Autodesk Inventor part; units mm, degrees
ref_plane "YZ Plane" through (0, 0, 0) normal (1, 0, 0) x (0, 1, 0)
ref_plane "XZ Plane" through (0, 0, 0) normal (0, 1, 0) x (-1, 0, 0)
ref_plane "XY Plane" through (0, 0, 0) normal (0, 0, 1) x (1, 0, 0)
sketch "Sketch6" plane through (0, 0, 0) normal (0, 1, 0) x (-1, 0, 0)
  line L0 (407.1, -490) -> (-407.1, -490)
  line L1 (-407.1, -490) -> (-407.1, 490)
  line L2 (-407.1, 490) -> (407.1, 490)
  line L3 (407.1, 490) -> (407.1, -490)
  line L4 (407.1, -490) -> (-407.1, 490) construction
  line L5 (-407.1, -490) -> (407.1, 490) construction
  point P0 (0, 0)
  dimension "d52" = 814.2
  dimension "d53" = 980
extrude "Plate2" add sketch "Sketch6" along normal blind 0.5
sketch "Sketch11" plane through (406.6, 0, -490) normal (1, 0, 0) x (0, 1, 0)
  line L0 (0, 980) -> (0, 0)
  line L1 (0, 0) -> (10, 0)
  line L2 (10, 0) -> (10, 980)
  line L3 (10, 980) -> (0, 980)
edge flange "Flange2" height 10 angle 90 thickness 0.5 bend radius 0.5 thickness toward (1, 0, 0) relief tear relief width 0.5 relief depth 0.25 edges at (407.1, 0.5, 0) wall of the first edge with corners at (406.6, 0, 490) (406.6, 0, -490) (406.6, 10, -490) (406.6, 10, 490)
bend "Bend3"
corner "Corner3"
sketch "Sketch12" plane through (407.1, 9.5, -490) normal (0, 1, 0) x (-1, 0, 0)
  line L0 (0, 980) -> (0, 0)
  line L1 (0, 0) -> (10, 0)
  line L2 (10, 0) -> (10, 980)
  line L3 (10, 980) -> (0, 980)
edge flange "Flange3" height 10 angle 90 thickness 0.5 bend radius 0.5 thickness toward (0, 1, 0) relief tear relief width 0.5 relief depth 0.25 edges at (406.6, 10, 0) wall of the first edge with corners at (407.1, 9.5, 490) (407.1, 9.5, -490) (397.1, 9.5, -490) (397.1, 9.5, 490)
bend "Bend4"
corner "Corner4"
sketch "Sketch13" plane through (-406.6, 0, 490) normal (-1, 0, 0) x (0, -1, 0)
  line L0 (0, -980) -> (0, 0)
  line L1 (0, 0) -> (-10, 0)
  line L2 (-10, 0) -> (-10, -980)
  line L3 (-10, -980) -> (0, -980)
edge flange "Flange4" height 10 angle 90 thickness 0.5 bend radius 0.5 thickness toward (-1, 0, 0) relief tear relief width 0.5 relief depth 0.25 edges at (-407.1, 0.5, 0) wall of the first edge with corners at (-406.6, 0, -490) (-406.6, 0, 490) (-406.6, 10, 490) (-406.6, 10, -490)
bend "Bend5"
corner "Corner5"
sketch "Sketch14" plane through (-407.1, 9.5, 490) normal (0, 1, 0) x (-1, 0, 0)
  line L0 (0, -980) -> (0, 0)
  line L1 (0, 0) -> (-10, 0)
  line L2 (-10, 0) -> (-10, -980)
  line L3 (-10, -980) -> (0, -980)
edge flange "Flange5" height 10 angle 90 thickness 0.5 bend radius 0.5 thickness toward (0, 1, 0) relief tear relief width 0.5 relief depth 0.25 edges at (-406.6, 10, 0) wall of the first edge with corners at (-407.1, 9.5, -490) (-407.1, 9.5, 490) (-397.1, 9.5, 490) (-397.1, 9.5, -490)
bend "Bend6"
corner "Corner6"
fillet "Corner Round1" radius 4 1 edges at (397.1, 9.75, 490)
fillet "Corner Round2" radius 4 1 edges at (397.1, 9.75, -490)
fillet "Corner Round3" radius 4 1 edges at (-397.1, 9.75, -490)
fillet "Corner Round4" radius 4 1 edges at (-397.1, 9.75, 490)
equation "\"d52\" = ЖАБРЫ_базовая_ширина - ЖАБРЫ_шаг_листов"
equation "\"d53\" = ЖАБРЫ_базовая_длина_кор_лист"
equation "\"d54\" = Thickness"
equation "\"d84\" = BendReliefWidth"
equation "\"d85\" = BendReliefDepth"
equation "\"d86\" = MinimumRemnant"
equation "\"d87\" = TransitionRadius"
equation "\"d90\" = BendRadius"
equation "\"d91\" = CornerReliefSize"
equation "\"d92\" = GapSize"
equation "\"d93\" = JacobiRadiusSize"
equation "\"d94\" = BendReliefWidth"
equation "\"d95\" = BendReliefDepth"
equation "\"d96\" = MinimumRemnant"
equation "\"d97\" = TransitionRadius"
equation "\"d100\" = BendRadius"
equation "\"d101\" = CornerReliefSize"
equation "\"d102\" = GapSize"
equation "\"d103\" = JacobiRadiusSize"
equation "\"d104\" = BendReliefWidth"
equation "\"d105\" = BendReliefDepth"
equation "\"d106\" = MinimumRemnant"
equation "\"d107\" = TransitionRadius"
equation "\"d110\" = BendRadius"
equation "\"d111\" = CornerReliefSize"
equation "\"d112\" = GapSize"
equation "\"d113\" = JacobiRadiusSize"
equation "\"d114\" = BendReliefWidth"
equation "\"d115\" = BendReliefDepth"
equation "\"d116\" = MinimumRemnant"
equation "\"d117\" = TransitionRadius"
equation "\"d120\" = BendRadius"
equation "\"d121\" = CornerReliefSize"
equation "\"d122\" = GapSize"
equation "\"d123\" = JacobiRadiusSize"
equation "\"BendRadius\" = Thickness"
equation "\"BendReliefWidth\" = Thickness"
equation "\"BendReliefDepth\" = 0.5 * Thickness"
equation "\"CornerReliefSize\" = 4 * Thickness"
equation "\"MinimumRemnant\" = 2 * Thickness"
equation "\"TransitionRadius\" = BendRadius"
equation "\"JacobiRadiusSize\" = BendRadius"
equation "\"GapSize\" = Thickness"
properties part number "MSC 805 SHEET GILLS" material "Stainless Steel"
Read the model definition and answer for the solid it produces. Units are mm, in the model's axes. Round coordinates to 2 decimals unless told otherwise and drop trailing zeros. Write each loop counter-clockwise with the first axis right and the second up, starting at its lowest first coordinate (ties: lowest second). Pieces come first, ordered by that corner, then holes. Notation, with made-up numbers: M 10,-36.5 L 26,-36.5 A36 ccw 26,2.5 Z; hole C 23,78.5 d6. An arc over 180 degrees is marked long. One line per item, written item: value.
Q1. Find section A-A on y = 3.75. Write down the section's boundary in (x, z), plus the area to 3 significant figures.
Data:
outline: M -407.1,-490 L -406.6,-490 L -406.6,490 L -407.1,490 Z; M 406.6,-490 L 407.1,-490 L 407.1,490 L 406.6,490 Z
area: 980 mm2
Q2. Find section C-C on x = 64. Write down the section's boundary in (y, z), plus the area to 3 significant figures.
Data:
outline: M 0,-490 L 0.5,-490 L 0.5,490 L 0,490 Z
area: 490 mm2
Q3. Find section B-B on z = -40. Write down the section's boundary in (x, y), plus the area to 3 significant figures.
Data:
outline: M -407.1,1 A1 ccw -406.1,0 L 406.1,0 A1 ccw 407.1,1 L 407.1,9 A1 ccw 406.1,10 L 397.1,10 L 397.1,9.5 L 406.1,9.5 A0.5 cw 406.6,9 L 406.6,1 A0.5 cw 406.1,0.5 L -406.1,0.5 A0.5 cw -406.6,1 L -406.6,9 A0.5 cw -406.1,9.5 L -397.1,9.5 L -397.1,10 L -406.1,10 A1 ccw -407.1,9 Z
area: 425 mm2
Q4. For a pull along X with two mould halves and no side action, classify faces 1 (the flat face through (6, 0, 7)), 2 (the flat face through (6, 0.5, 7)) as +X half, -X half, draft (parallel to the pull), parting line (faces both ways), or undercut.
Data:
face 1: draft
face 2: undercut
Q5. A flat-ended cylindrical pin translates along its axis: pin 1 Ø1 at (x, y) = (-41, 1.5) entering from +Z. Find the tip coordinate at first contact, or state that the pin passes through.
Data:
pin 1: through
Q6. Straight lines are drawn through the part: line 1 (X direction, y = 3, z = -213.5); line 2 (Y direction, x = 98, z = -403); line 3 (X direction, y = 9.25, z = 440). For each, find the intervals that lie inside material, in ascending order. Write a range as [from, to].
Data:
line 1: [-407.1, -406.6], [406.6, 407.1]
line 2: [0, 0.5]
line 3: [-407.07, -406.53], [406.53, 407.07]
